For this review, use the dimensioned drawing (mm, ordinates from the lowest corner) and the shaded views. A direction names the side the tool comes from. Coordinates: 2 decimals unless noted, no trailing zeros. Loops run counter-clockwise (first coordinate to the right, second up) from the corner with the lowest first, then second, coordinate; pieces in that order, holes last.
1. Take a section at A-A, the plane z = 11. State the section outline as (x, y) points (1 decimal).
2. Take a section at B-B, the plane y = 20. State the section outline as (x, z) points, then the cut area to 3 significant figures.
3. Machinability: for the marked faces 1, 2 and 3, which of the approach directions +Z, -Z, +X, -X, +Y, -Y give a long, thin tool a straight path to every point of the face, cutting with its end or side? Answer none if there is none.
4. Mouldability with a two-part tool opening along Y and no side actions: class the marked faces 4, 5 and 6 as pulls with the +Y half, pulls with the -Y half, needs draft (parallel to the pull), parting line crosses it, or undercut.
5. Clearance check with flat-ended pins moving along their axes: P1, Ø6, axis at y = 9, z = 5, coming from the +X side; P2, Ø5.5, axis at y = 25, z = 5.5, coming from the -X side; P3, Ø2.5, axis at x = 30.5, z = 6.5, coming from the +Y side. State where each tip first meets the part, or that it passes through.
6. Take a section at C-C, the plane x = 9. State the section outline as (y, z) points (1 decimal), then the cut area to 3 significant figures.
7. Take a section at D-D, the plane y = 13. State the section outline as (x, z) points.
8. To check wall thickness, follow probe 1 along X at (y, z) = (20, 6); probe 2 along Z at (x, y) = (2.5, 21) (1 decimal); probe 3 along X at (y, z) = (11, 10). State the ranges of each line that lie inside material, in increasing order.
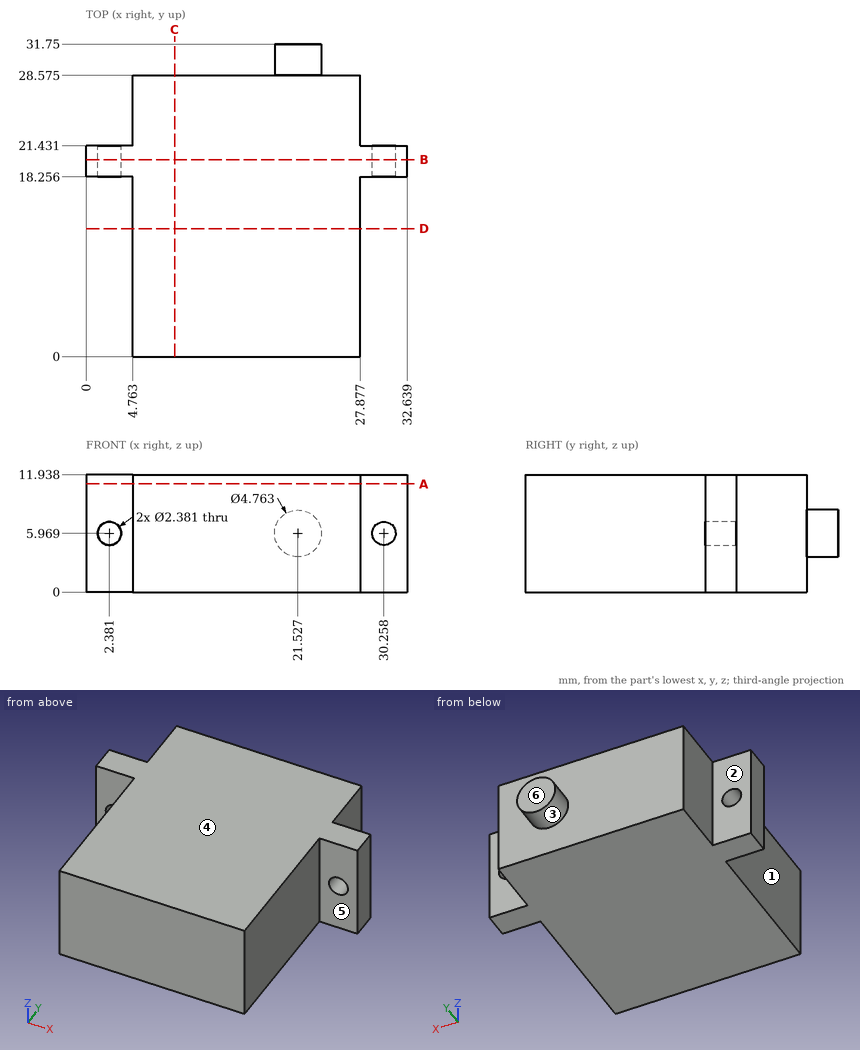
Results list:
1. outline: (0, 18.3) - (4.8, 18.3) - (4.8, 0) - (27.9, 0) - (27.9, 18.3) - (32.6, 18.3) - (32.6, 21.4) - (27.9, 21.4) - (27.9, 28.6) - (4.8, 28.6) - (4.8, 21.4) - (0, 21.4) - close
2. outline: (0, 0) - (32.64, 0) - (32.64, 11.94) - (0, 11.94) - close; hole circle Ø2.38 at (2.38, 5.97); hole circle Ø2.38 at (30.26, 5.97)
2. area: 381 mm2
3. face 1: +Z, -Z, -X, -Y
3. face 2: +Z, -Z, -X, +Y
3. face 3: +Y
4. face 4: needs draft
4. face 5: pulls with the -Y half
4. face 6: pulls with the +Y half
5. P1: stops at x = 27.88
5. P2: stops at x = 4.76
5. P3: stops at y = 21.43
6. outline: (0, 0) - (28.6, 0) - (28.6, 11.9) - (0, 11.9) - close
6. area: 341 mm2
7. outline: (4.76, 0) - (27.88, 0) - (27.88, 11.94) - (4.76, 11.94) - close
8. probe 1: x = 0 to 1.19, 3.57 to 29.07, 31.45 to 32.64
8. probe 2: z = 0 to 4.8, 7.2 to 11.9
8. probe 3: x = 4.76 to 27.88
